Source: CAD feature listing. Evaluate the final solid. Frame: model axes, mm. A direction names the side the tool comes from. Round coordinates to 2 decimals unless told otherwise and drop trailing zeros. Order: outer loops, then holes, each group sorted by start corner. A loop starts at its lowest first (then second) coordinate and runs counter-clockwise, first axis right, second up. Notation, with made-up numbers: (-19, 43) - (31, 43) arc R18 ccw to (31, 71) - close; hole circle Ø3 at (-16, 77.25). An arc over 180 degrees is marked (long way). Use one line per item in the form item = value. Start each with the question number.
Q1. Ray query, line 1 (X direction, y = -40.5, z = 2); line 2 (Y direction, x = -9.75, z = -5.5); line 3 (Z direction, x = 10.75, y = -13.5). Return the intervals inside material, ascending. Write a range as [from, to].
Q2. Draft query along X for faces 4 (the flat face through (0, 3, 0)), 5 (the cylindrical face through (-4.58, 1.48, 0.3)), 6 (the flat face through (-10, -31, 0)), 7 (the flat face through (-13, -30, 0)). Return one class per face: released by +X, released by -X, zero draft, split by the parting line, or undercut.
Q3. Pin query (flat end, axial travel): pin 1 Ø0.9 at (x, z) = (-11, 2.5) entering from -Y; pin 2 Ø5 at (y, z) = (-60, -11) entering from -X; pin 3 Ø3.5 at (x, z) = (11.5, 14) entering from +Y. Return the tip coordinate at first contact, or that it passes through.
Q4. Cut plane B-B, the plane z = 0. Give the number of separate pieces and of enclosed holes in the cut face, and give its area (3 significant figures).
Q5. Cut plane D-D, the plane x = -3.25. Return the cut outline in (y, z), and give its area (3 significant figures).
Q6. Cut plane C-C, the plane y = -17. Return the cut outline in (x, z) (3 decimals).
Q7. Cut plane A-A, the plane y = -26. Return the cut outline in (x, z), and give its area (3 significant figures).
Q8. Set-up query: faces 1 (the flat face through (12, -58, -11)), 2 (the flat face through (12, -69, 12)), 3 (the flat face through (0, 0, 0)). Return all of +Z, -Z, +X, -X, +Y, -Y with unobstructed straight access to the full face (end or side cutting, diameter ignored); none if empty.
from build123d import *

# Parameters (mm, degrees)
SKETCH2_W           = 26
SKETCH2_H           = 12
BOSS_EXTRUDE1_DEPTH = 3
SKETCH3_R           = 1
CUT_EXTRUDE1_DEPTH  = 10
SKETCH4_W           = 3
SKETCH4_H           = 12
BOSS_EXTRUDE2_DEPTH = 75
SKETCH5_R           = 1.425
CUT_EXTRUDE2_DEPTH  = 30
LPATTERN1_COUNT     = 2
LPATTERN1_PITCH     = 35
BOSS_EXTRUDE3_DEPTH = 3
SKETCH7_R           = 1
CUT_EXTRUDE3_DEPTH  = 3
SKETCH8_W           = 12
SKETCH8_H           = 12
CUT_EXTRUDE4_DEPTH  = 27


with BuildPart() as part:
    # Sketch2 → Boss-Extrude1 (new body)
    with BuildSketch(Plane(origin=(0, 0, 0), x_dir=(1, 0, 0), z_dir=(0, 1, 0))):
        Rectangle(SKETCH2_W, SKETCH2_H)
    extrude(amount=BOSS_EXTRUDE1_DEPTH)

    # Sketch3 → Cut-Extrude1 (cut)
    with BuildSketch(Plane.XZ):
        with Locations((-5.535, 0)):
            Circle(SKETCH3_R)
        with Locations((5.535, 0)):
            Circle(SKETCH3_R)
    extrude(amount=-CUT_EXTRUDE1_DEPTH, mode=Mode.SUBTRACT)

    # Sketch4 → Boss-Extrude2 (add)
    with BuildSketch(Plane.XZ):
        with Locations((-11.5, 0)):
            Rectangle(SKETCH4_W, SKETCH4_H)
    boss_extrude2 = extrude(amount=BOSS_EXTRUDE2_DEPTH)

    # Mirror1: Boss-Extrude2 across plane
    add(boss_extrude2.mirror(Plane(origin=(0, 0, 0), x_dir=(0, 0, 1), z_dir=(1, 0, 0))))

    # Sketch5 → Cut-Extrude2 (cut)
    with BuildSketch(Plane.ZY.offset(13)):
        with Locations((0, -17)):
            Circle(SKETCH5_R)
    cut_extrude2 = extrude(amount=-CUT_EXTRUDE2_DEPTH, mode=Mode.SUBTRACT)

    # LPattern1: Cut-Extrude2 ×2
    with Locations(*[(0, -i * LPATTERN1_PITCH, 0) for i in range(1, LPATTERN1_COUNT)]):
        add(cut_extrude2, mode=Mode.SUBTRACT)

    # Sketch6 → Boss-Extrude3 (add)
    with BuildSketch(Plane(origin=(13, 0, 0), x_dir=(0, 0, -1), z_dir=(1, 0, 0))):
        Polygon((-6, -58), (-17, -58), (-17, -63), (-17, -75), (-12, -75), (-12, -63), (-6, -63), align=None)
    boss_extrude3 = extrude(amount=-BOSS_EXTRUDE3_DEPTH)

    # Mirror2: Boss-Extrude3 across plane
    add(boss_extrude3.mirror(Plane.XY))

    # Sketch7 → Cut-Extrude3 (cut)
    with BuildSketch(Plane(origin=(13, 0, 0), x_dir=(0, 0, -1), z_dir=(1, 0, 0))):
        with Locations((-13.625, -69.526287367)):
            Circle(SKETCH7_R)
    cut_extrude3 = extrude(amount=-CUT_EXTRUDE3_DEPTH, mode=Mode.SUBTRACT)

    # Mirror3: Cut-Extrude3 across plane
    add(cut_extrude3.mirror(Plane.XY), mode=Mode.SUBTRACT)

    # Sketch8 → Cut-Extrude4 (cut, through all)
    with BuildSketch(Plane(origin=(13, 0, 0), x_dir=(0, 0, -1), z_dir=(1, 0, 0))):
        with Locations((0, -69)):
            Rectangle(SKETCH8_W, SKETCH8_H)
    extrude(amount=-CUT_EXTRUDE4_DEPTH, mode=Mode.SUBTRACT)


solid = part.part
Completed:
q1.line_1 = [-13, -10], [10, 13]
q1.line_2 = [0, 3]
q1.line_3 = [-6, 6]
q2.face_4 = zero draft
q2.face_5 = undercut
q2.face_6 = undercut
q2.face_7 = released by -X
q3.pin_1 = -63
q3.pin_2 = 10
q3.pin_3 = -58
q4.separate_pieces = 7
q4.enclosed_holes = 0
q4.area = 410 mm2
q5.outline = (0, -6) - (3, -6) - (3, 6) - (0, 6) - close
q5.area = 36.0 mm2
q6.outline = (-13, -6) - (-10, -6) - (-10, -1.425) - (-13, -1.425) - close; (-13, 1.425) - (-10, 1.425) - (-10, 6) - (-13, 6) - close; (10, -6) - (13, -6) - (13, -1.425) - (10, -1.425) - close; (10, 1.425) - (13, 1.425) - (13, 6) - (10, 6) - close
q7.outline = (-13, -6) - (-10, -6) - (-10, 6) - (-13, 6) - close; (10, -6) - (13, -6) - (13, 6) - (10, 6) - close
q7.area = 72.0 mm2
q8.face_1 = -Z, +X, -X, +Y
q8.face_2 = +X, -X, -Y
q8.face_3 = +Z, -Z, -Y
